Build history of the part. All positions in model axes, mm. Face numbers are marked on the shaded views. A direction names the side the tool comes from. Give positions to 0.01 mm unless a question says otherwise; leave off trailing zeros. Write each loop counter-clockwise with the first axis right and the second up, starting at its lowest first coordinate (ties: lowest second). Pieces come first, ordered by that corner, then holes. Notation, with made-up numbers: M 87.5,89.25 L 111.5,89.25 A23 cw 111.5,98.25 Z; hole C -14,14.25 d1. An arc over 180 degrees is marked long. Return JSON: item names as keys, results as strings. Group by question number.
Q1. Tool access for the marked faces 1 and 2: list every direction of +Z, -Z, +X, -X, +Y, -Y with a clear straight run to the whole face (end or side of a thin tool).
Q2. Pull direction Y, two halves, no side cores. Call the marked faces 3, 4, 5 and 6: +Y half, -Y half, draft (parallel to the pull), parting line (faces both ways), or undercut.
Q3. Band-saw the part on B-B, the plane x = -56. Give the cut face in (y, z), then the cut area to 3 significant figures.
Q4. Band-saw the part on C-C, the plane y = 29.5. Give the cut face in (x, z).
Q5. Band-saw the part on A-A, the plane z = 5.5. Give the cut face in (x, y).
Q6. Wall check: probe 1 along X at (y, z) = (15.5, 6.25); probe 2 along Y at (x, z) = (-61, 7.75); probe 3 along Z at (x, y) = (-57, 7.5). Give the ranges that are in metal, low to high.
from build123d import *

# Parameters (mm, degrees)
F0_W     = 66
F0_H     = 55
F1_DEPTH = 10
F2_T     = -2
F3_R     = 3
F4_R     = 3
F5_R     = 3
F6_R     = 3


with BuildPart() as f1:
    # F0 (on Top) → F1 (new body)
    with BuildSketch(Plane.XY):
        with Locations((-33, 27.5)):
            Rectangle(F0_W, F0_H)
    extrude(amount=F1_DEPTH)

    # F2
    f2_openings = [f1.faces().sort_by_distance(p)[0] for p in [
        (-33, 27.5, 10),
    ]]
    offset(amount=F2_T, openings=f2_openings)

    # F3
    f3_edges = [f1.edges().sort_by_distance(p)[0] for p in [
        (0, 55, 5),
    ]]
    fillet(f3_edges, radius=F3_R)

    # F4
    f4_edges = [f1.edges().sort_by_distance(p)[0] for p in [
        (0, 0, 5),
    ]]
    fillet(f4_edges, radius=F4_R)

    # F5
    f5_edges = [f1.edges().sort_by_distance(p)[0] for p in [
        (-66, 55, 5),
    ]]
    fillet(f5_edges, radius=F5_R)

    # F6
    f6_edges = [f1.edges().sort_by_distance(p)[0] for p in [
        (-66, 0, 5),
    ]]
    fillet(f6_edges, radius=F6_R)


solid = f1.part
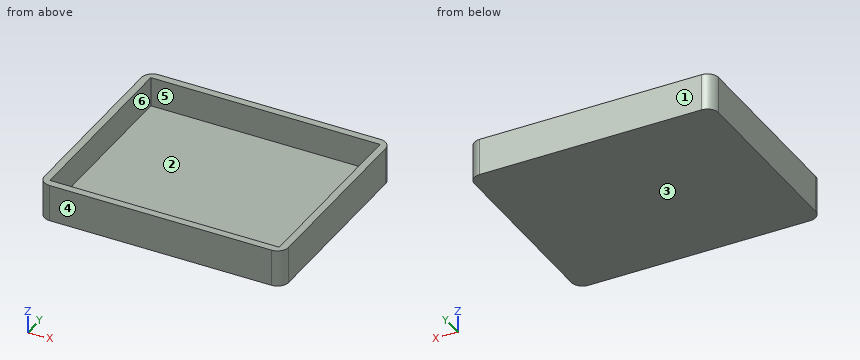
From the geometry:
{
 "1": {"face 1": "+Z, -Z, +X, -X, +Y", "face 2": "+Z"},
 "2": {"face 3": "draft", "face 4": "-Y half", "face 5": "undercut", "face 6": "undercut"},
 "3": {"outline": "M 0,0 L 55,0 L 55,10 L 53,10 L 53,2 L 2,2 L 2,10 L 0,10 Z", "area": "142 mm^2"},
 "4": {"outline": "M -66,0 L 0,0 L 0,10 L -2,10 L -2,2 L -64,2 L -64,10 L -66,10 Z"},
 "5": {"outline": "M -66,3 A3 ccw -63,0 L -3,0 A3 ccw 0,3 L 0,52 A3 ccw -3,55 L -63,55 A3 ccw -66,52 Z; hole M -64,2 L -2,2 L -2,53 L -64,53 Z"},
 "6": {"probe 1": "x = -66 to -64, -2 to 0", "probe 2": "y = 0 to 2, 53 to 55", "probe 3": "z = 0 to 2"}
}
